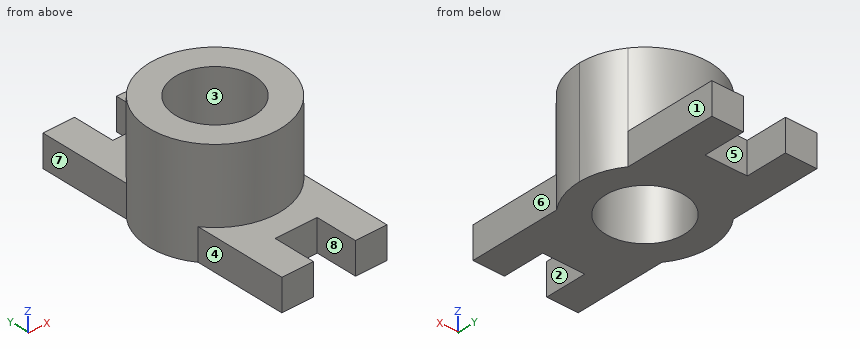
from build123d import *

# Parameters (mm, degrees)
F0_R     = 15
F1_DEPTH = 40
F2_DEPTH = 12


with BuildPart() as f1:
    # F0 (on Top) → F1 (new body)
    with BuildSketch(Plane.XY):
        with BuildLine():
            ThreePointArc((-23.643522, 45.745022), (-28.643522, 30.745022), (-23.643522, 15.745022))
            ThreePointArc((-23.643522, 15.745022), (-3.643522, 5.745022), (16.356478, 15.745022))
            ThreePointArc((16.356478, 15.745022), (20.07356, 22.839328), (21.356478, 30.745022))
            ThreePointArc((21.356478, 30.745022), (20.07356, 38.650717), (16.356478, 45.745022))
            ThreePointArc((16.356478, 45.745022), (-3.643522, 55.745022), (-23.643522, 45.745022))
        make_face()
        with Locations((-3.643522, 30.745022)):
            Circle(F0_R, mode=Mode.SUBTRACT)
    extrude(amount=F1_DEPTH)

    # F0 (on Top) → F2 (join)
    with BuildSketch(Plane.XY):
        with BuildLine():
            Line((-23.643522, 15.745022), (-23.643522, -19.254978))
            Line((-23.643522, -19.254978), (-11.643522, -19.254978))
            Line((-11.643522, -19.254978), (-11.643522, -3.254978))
            Line((-11.643522, -3.254978), (4.356478, -3.254978))
            Line((4.356478, -3.254978), (4.356478, -19.254978))
            Line((4.356478, -19.254978), (16.356478, -19.254978))
            Line((16.356478, -19.254978), (16.356478, 15.745022))
            ThreePointArc((16.356478, 15.745022), (-3.643522, 5.745022), (-23.643522, 15.745022))
        make_face()
        with BuildLine():
            Line((-23.643522, 80.745022), (-23.643522, 45.745022))
            ThreePointArc((-23.643522, 45.745022), (-3.643522, 55.745022), (16.356478, 45.745022))
            Line((16.356478, 45.745022), (16.356478, 80.745022))
            Line((16.356478, 80.745022), (4.356478, 80.745022))
            Line((4.356478, 80.745022), (4.356478, 64.745022))
            Line((4.356478, 64.745022), (-11.643522, 64.745022))
            Line((-11.643522, 64.745022), (-11.643522, 80.745022))
            Line((-11.643522, 80.745022), (-23.643522, 80.745022))
        make_face()
    extrude(amount=F2_DEPTH)


solid = f1.part
Can you work these out from the model? Positions are in its coordinate system, mm. Face numbers are marked on the shaded views. A direction names the side the tool comes from. Round coordinates to 2 decimals unless told otherwise and drop trailing zeros. Order: outer loops, then holes, each group sorted by start corner. A loop starts at its lowest first (then second) coordinate and runs counter-clockwise, first axis right, second up. Notation, with made-up numbers: (30.5, 28) - (58.5, 28) arc R32 cw to (58.5, 59) - close; hole circle Ø4 at (-5, 87). An arc over 180 degrees is marked (long way). Answer in a Markdown table with one row per item.
(1) Suppose I cut it at A-A, the plane y = 72.5. Please give me the cut outline in (x, z).
From the geometry:
| item | result |
|---|---|
| outline | (-23.64, 0) - (-11.64, 0) - (-11.64, 12) - (-23.64, 12) - close; (4.36, 0) - (16.36, 0) - (16.36, 12) - (4.36, 12) - close |
(2) Which directions (+Z, -Z, +X, -X, +Y, -Y) give clear straight access to the entire face, cutting with the end or side of a thin tool? Please do the marked faces 5, 6, 7 and 8.
From the geometry:
| item | result |
|---|---|
| face 5 | +Z, -Z, +Y |
| face 6 | +Z, -Z, +X, -Y |
| face 7 | +Z, -Z, -X, +Y |
| face 8 | +Z, -Z, -Y |
(3) If we mould it in two halves opening along X, with no side actions, what happens to the marked faces 1, 2, 3 and 4? For each: released by +X, released by -X, zero draft, split by the parting line, or undercut.
From the geometry:
| item | result |
|---|---|
| face 1 | released by +X |
| face 2 | undercut |
| face 3 | undercut |
| face 4 | released by -X |
(4) Suppose I cut it at C-C, the plane x = 5.5. Please give me the cut outline in (y, z).
From the geometry:
| item | result |
|---|---|
| outline | (-19.25, 0) - (18.85, 0) - (18.85, 40) - (7.48, 40) - (7.48, 12) - (-19.25, 12) - close; (42.64, 0) - (80.75, 0) - (80.75, 12) - (54.01, 12) - (54.01, 40) - (42.64, 40) - close |
(5) For P1, Ø3, axis at x = -1.5, z = 29.5, coming from the -Y side; P2, Ø4, axis at x = 10.5, z = 22, coming from the -Y side; P3, Ø6, axis at x = -18.5, z = 30, coming from the +Y side, each with a flat end and sliding along its axis, tell me the tip position at first contact or that it passes through.
From the geometry:
| item | result |
|---|---|
| P1 | stops at y = 5.75 |
| P2 | stops at y = 8.89 |
| P3 | stops at y = 52.75 |
(6) Please list where these lines run through material, in increasing order: L1, parallel to X at y = 76, z = 3; L2, parallel to Z at x = -9.5, y = -1; L3, parallel to Y at x = 4, z = 9.5. Write a range as from..to.
From the geometry:
| item | result |
|---|---|
| L1 | x = -23.64..-11.64, 4.36..16.36 |
| L2 | z = 0..12 |
| L3 | y = -3.25..17.84, 43.65..64.75 |
(7) Suppose I cut it at B-B, the plane z = 6. Please give me the cut outline in (x, y).
From the geometry:
| item | result |
|---|---|
| outline | (-23.64, -19.25) - (-11.64, -19.25) - (-11.64, -3.25) - (4.36, -3.25) - (4.36, -19.25) - (16.36, -19.25) - (16.36, 15.75) arc R25 ccw to (21.36, 30.75) arc R25 ccw to (16.36, 45.75) - (16.36, 80.75) - (4.36, 80.75) - (4.36, 64.75) - (-11.64, 64.75) - (-11.64, 80.75) - (-23.64, 80.75) - (-23.64, 45.75) arc R25 ccw to (-23.64, 15.75) - close; hole circle Ø30 at (-3.64, 30.75) |
(8) Suppose I cut it at D-D, the plane x = -4. Please give me the cut outline in (y, z), plus the area to 3 significant figures.
From the geometry:
| item | result |
|---|---|
| outline | (-3.25, 0) - (15.75, 0) - (15.75, 40) - (5.75, 40) - (5.75, 12) - (-3.25, 12) - close; (45.74, 0) - (64.75, 0) - (64.75, 12) - (55.74, 12) - (55.74, 40) - (45.74, 40) - close |
| area | 1,020 mm2 |
